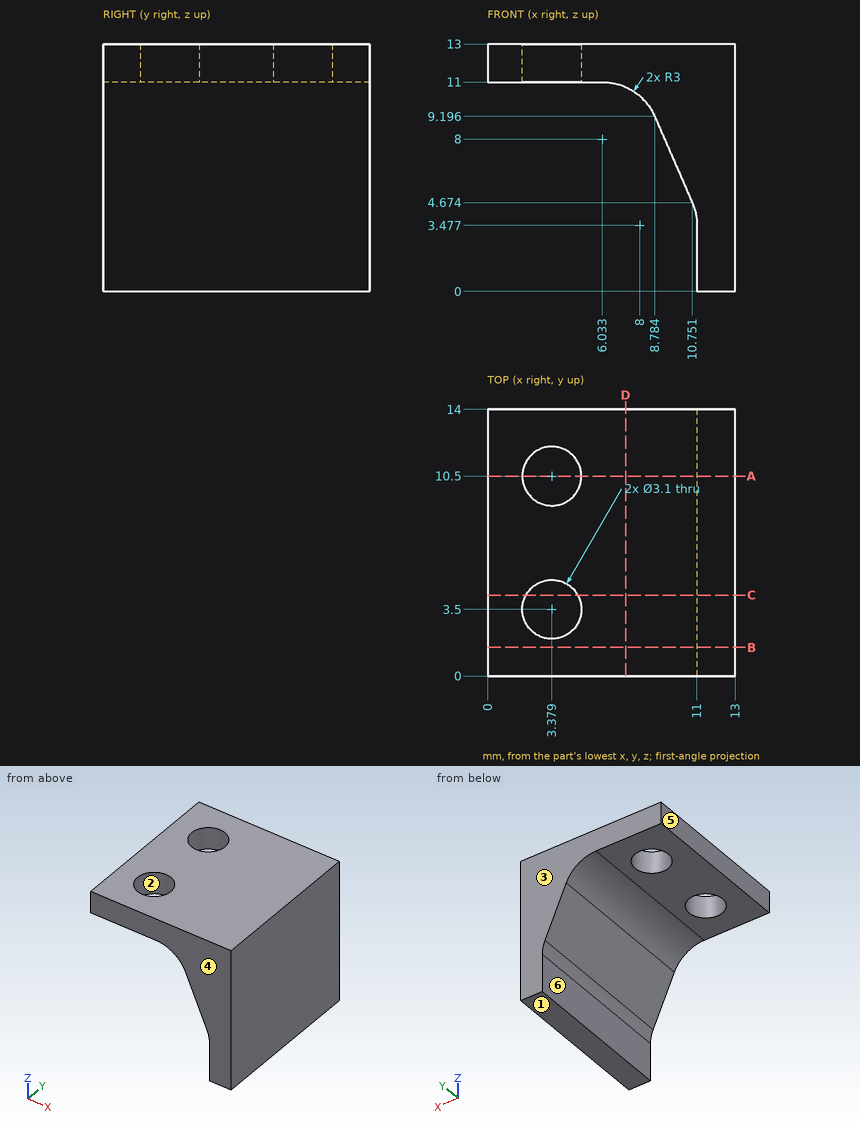
Input: dimensioned drawing with shaded views. Units: mm. Origin: part minimum x, y, z. A direction names the side the tool comes from. Coordinates: 2 decimals unless noted, no trailing zeros. Write each loop counter-clockwise with the first axis right and the second up, starting at its lowest first coordinate (ties: lowest second). Pieces come first, ordered by that corner, then holes. Notation, with made-up numbers: M 74,-14.5 L 88,-14.5 A23 ccw 88,3.5 Z; hole C 88,-22.75 d1. An arc over 180 degrees is marked long. Answer as a JSON object with one key per item and string values. Group by question number.
(1) Section D-D on x = 7.25. Output: boundary loops of the cut face in (y, z).
(2) Contact query for flat-ended pins moving along their axis: P1, Ø6.5, axis at x = 4.5, y = 8, coming from the -Z side; P2, Ø3, axis at x = 7.5, z = 10, coming from the -Y side; P3, Ø1, axis at y = 5, z = 9, coming from the -X side; P4, Ø3, axis at y = 4, z = 1, coming from the -X side. Output: stop coordinate, or through.
(3) Ray query, line 1 along X through (y, z) = (10.5, 11.9); line 2 along Y through (x, z) = (2.75, 11.75); line 3 along Z through (x, y) = (3.5, 8.25). Return the intervals inside material, ascending. Write a range as [from, to].
(4) Mould query, pull axis Y, two halves, no side actions, for the marked faces 1, 2, 3 and 4. Classes: pulls with the +Y half, pulls with the -Y half, needs draft (parallel to the pull), parting line crosses it, or undercut.
(5) Set-up query: the marked faces 5 and 6. Return all of +Z, -Z, +X, -X, +Y, -Y with unobstructed straight access to the full face (end or side cutting, diameter ignored); none if empty.
(6) Section A-A on y = 10.5. Output: boundary loops of the cut face in (x, z) (1 decimal).
(7) Section C-C on y = 4.25. Output: boundary loops of the cut face in (x, z) (1 decimal).
(8) Section B-B on y = 1.5. Output: boundary loops of the cut face in (x, z) (1 decimal).
Result set:
{
 "1": {"outline": "M 0,10.74 L 14,10.74 L 14,13 L 0,13 Z"},
 "2": {"P1": "stops at z = 10.46", "P2": "stops at y = 0", "P3": "stops at x = 8.63", "P4": "stops at x = 11"},
 "3": {"line 1": "x = [0, 1.83], [4.93, 13]", "line 2": "y = [0, 2.08], [4.92, 9.08], [11.92, 14]", "line 3": "z = [11, 13]"},
 "4": {"face 1": "needs draft", "face 2": "undercut", "face 3": "pulls with the +Y half", "face 4": "pulls with the -Y half"},
 "5": {"face 5": "+Z, -Z, -X, +Y, -Y", "face 6": "-Z, -X, +Y, -Y"},
 "6": {"outline": "M 0,11 L 1.8,11 L 1.8,13 L 0,13 Z; M 4.9,11 L 6,11 A3 cw 8.8,9.2 L 10.8,4.7 A3 cw 11,3.5 L 11,0 L 13,0 L 13,13 L 4.9,13 Z"},
 "7": {"outline": "M 0,11 L 2,11 L 2,13 L 0,13 Z; M 4.7,11 L 6,11 A3 cw 8.8,9.2 L 10.8,4.7 A3 cw 11,3.5 L 11,0 L 13,0 L 13,13 L 4.7,13 Z"},
 "8": {"outline": "M 0,11 L 6,11 A3 cw 8.8,9.2 L 10.8,4.7 A3 cw 11,3.5 L 11,0 L 13,0 L 13,13 L 0,13 Z"}
}
